from build123d import *

# Parameters (mm, degrees)
F0_R     = 10
F1_DEPTH = 2
F2_R     = 6
F3_DEPTH = 0.45
F4_R     = 5.05
F5_DEPTH = 2
F6_SIZE  = 0.25
F8_SIZE  = 0.5


# Not quite as in the source:
# - a fillet or chamfer that OpenCascade refuses, or shapes differently, is made with other operations: its cross-section is extruded or revolved along the edge and cut away or added


with BuildPart() as f1:
    # F0 (on Top) → F1 (new body)
    with BuildSketch(Plane.XY):
        Circle(F0_R)
    extrude(amount=F1_DEPTH)

    # F2 (on face) → F3 (join)
    with BuildSketch(Plane.XY.offset(2)):
        Circle(F2_R)
    extrude(amount=F3_DEPTH)

    # F4 (on face) → F5 (join)
    with BuildSketch(Plane.XY.offset(2.45)):
        Circle(F4_R)
    extrude(amount=F5_DEPTH)

    # F6
    f6_edges = [f1.edges().sort_by_distance(p)[0] for p in [
        (-5.05, 0, 4.45),
    ]]
    chamfer(f6_edges, length=F6_SIZE)

    # F7: chamfer of 0.5 on 1 edges, made by hand


with BuildPart() as f7_tool2:
    # F7_s3 → F7_t4 (revolve)
    with BuildSketch(Plane.XZ):
        Polygon((5.5, 2.45), (6, 1.95), (6, 2.45), align=None)
    revolve(axis=Axis((0, 0, 2.45), (0, 0, 1)))

    split(bisect_by=Plane.XY.offset(2), keep=Keep.TOP)


with BuildPart() as f1_1:
    add(f1.part)

    # F7_t1: cut F7_tool2
    add(f7_tool2.part, mode=Mode.SUBTRACT)

    # F8
    f8_edges = [f1_1.edges().sort_by_distance(p)[0] for p in [
        (-10, 0, 0),
        (-10, 0, 2),
    ]]
    chamfer(f8_edges, length=F8_SIZE)


solid = f1_1.part
Design review of the part built by this model. Coordinates are the model's own, in mm. A direction names the side the tool comes from. Round coordinates to 2 decimals unless told otherwise and drop trailing zeros. Loops run counter-clockwise (first coordinate to the right, second up) from the corner with the lowest first, then second, coordinate; pieces in that order, holes last. Notation, with made-up numbers: (-34.5, -27.5) - (-26.5, -27.5) arc R25 ccw to (-26.5, -3.5) - close; hole circle Ø5 at (43.25, 79). An arc over 180 degrees is marked (long way). One line per question, with ' | ' between items.
1. We need section D-D, the plane z = 0.8. State the section outline as (x, y) points, and give its area (3 significant figures).
Results are:
outline: circle Ø20 at (0, 0) | area: 314 mm²
2. For L1, parallel to Z at x = -4.5, y = -4.75; L2, parallel to X at y = 8, z = 0.6; L3, parallel to Y at x = 1.75, z = 0.9, list the stretches that pass through material, from the lowest coordinate up. Write a range as [from, to].
Results are:
L1: z = [0, 2] | L2: x = [-6, 6] | L3: y = [-9.85, 9.85]
3. Clearance check with flat-ended pins moving along their axes: P1, Ø1.5, axis at x = 7, z = 1, coming from the +Y side; P2, Ø2, axis at x = 7.5, z = 2, coming from the +Y side; P3, Ø1.5, axis at x = 8, z = 3, coming from the -Y side; P4, Ø2, axis at x = -2, z = 2.5, coming from the -Y side. State where each tip first meets the part, or that it passes through.
Results are:
P1: stops at y = 7.81 | P2: stops at y = 7.48 | P3: passes through | P4: stops at y = -9.82
4. We need section A-A, the plane y = 0. State the section outline as (x, z) points, and give its area (3 significant figures).
Results are:
outline: (-10, 0.5) - (-9.5, 0) - (9.5, 0) - (10, 0.5) - (10, 1.5) - (9.5, 2) - (5.95, 2) - (5.5, 2.45) - (5.05, 2.45) - (5.05, 4.2) - (4.8, 4.45) - (-4.8, 4.45) - (-5.05, 4.2) - (-5.05, 2.45) - (-5.5, 2.45) - (-5.95, 2) - (-9.5, 2) - (-10, 1.5) - close | area: 64.8 mm²
5. For faces 1 (the face through (4.817, 1.517, 3.313)), 2 (the face through (0, 0, 0)), list the 3-axis set-ups (+Z, -Z, +X, -X, +Y, -Y) from which the entire face can be reached by the end or side of a thin tool; tool diameter is ignored.
Results are:
face 1: +Z | face 2: -Z, +X, -X, +Y, -Y
6. We need section C-C, the plane z = 3.3. State the section outline as (x, y) points.
Results are:
outline: circle Ø10.1 at (0, 0)
